The figure shows three views and two pictorial views of one solid part (mm, origin at its lowest corner). Answer the questions. Give positions to 0.01 mm unless a question says otherwise; leave off trailing zeros. Order: outer loops, then holes, each group sorted by start corner. A loop starts at its lowest first (then second) coordinate and runs counter-clockwise, first axis right, second up. Notation, with made-up numbers: (-4.75, 12.5) -> (36.25, 12.5) arc R24 cw to (36.25, 51.5) -> close; hole circle Ø1 at (49, 73). An arc over 180 degrees is marked (long way). One line per item, written item: value. Start each with the question number.
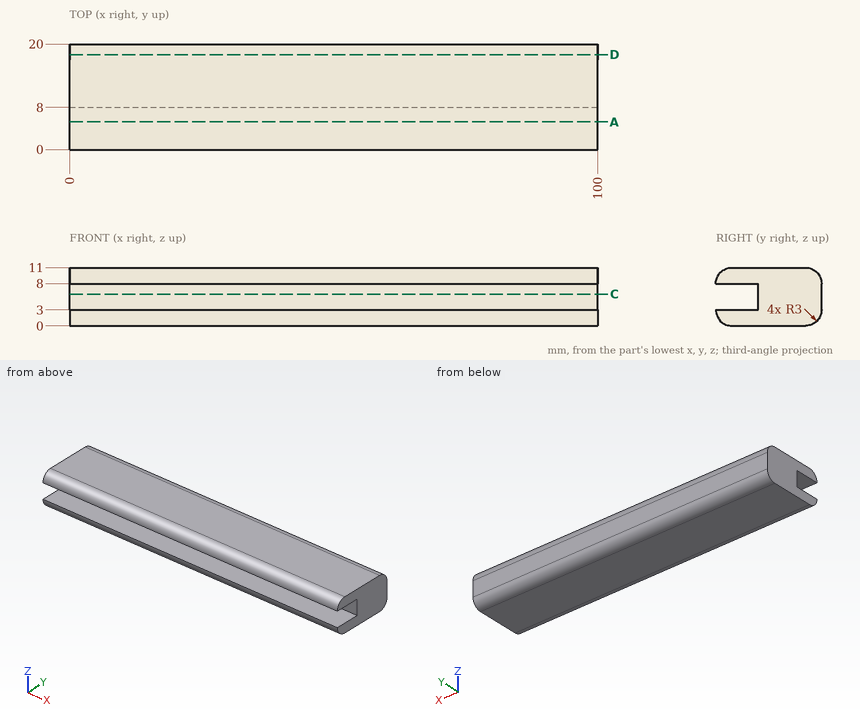
Item 1: Find section C-C on z = 6. Write down the section's boundary in (x, y).
Item 2: Find the intervals of material crossed by line 1 (Z direction, x = 82, y = 7.5); line 2 (Y direction, x = 31, z = 3.25); line 3 (Y direction, x = 52, z = 2.75), in increasing order. Write a range as from..to.
Item 3: Find section D-D on y = 18. Write down the section's boundary in (x, z).
Item 4: Find section A-A on y = 5.25. Write down the section's boundary in (x, z).
Checks:
1. outline: (0, 8) -> (100, 8) -> (100, 20) -> (0, 20) -> close
2. line 1: 0..3, 8..11
2. line 2: 8..20
2. line 3: 0.01..19.99
3. outline: (0, 0.17) -> (100, 0.17) -> (100, 10.83) -> (0, 10.83) -> close
4. outline: (0, 0) -> (100, 0) -> (100, 3) -> (0, 3) -> close; (0, 8) -> (100, 8) -> (100, 11) -> (0, 11) -> close
